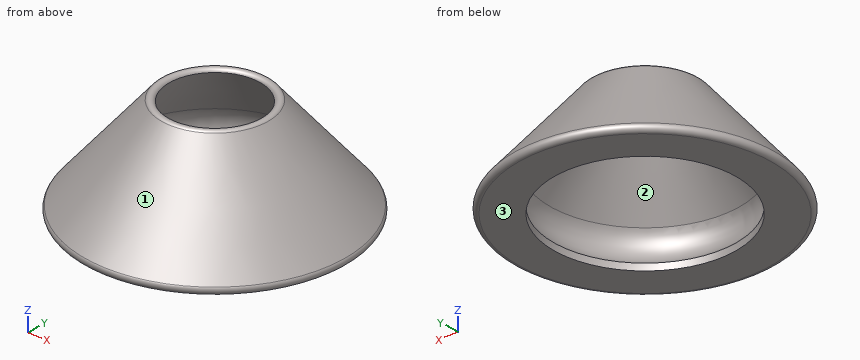
```python
from build123d import *


# Not quite as in the source:
# - a fillet or chamfer that OpenCascade refuses, or shapes differently, is made with other operations: its cross-section is extruded or revolved along the edge and cut away or added


with BuildPart() as f1:
    # F0 (on Front) → F1 (revolve)
    with BuildSketch(Plane.XZ):
        Polygon((20, 1.5), (20, 0), (30, 0), (10, 23.8350718519), (10, 21.5014861116), (26.7832396192, 1.5), align=None)
    revolve(axis=Axis((0, 0, 12.1238185093), (0, 0, 1)))

    # F2: fillet of radius 5 on 1 edges, made by hand

    # F2_s1 → F2_t2 (revolve)
    with BuildSketch(Plane.XZ):
        with BuildLine():
            ThreePointArc((20.7691072795, 8.6673638222), (21.9103444044, 4.9199541008), (20, 1.5))
            Line((20, 1.5), (20.0612222987, 1.4209314845))
            ThreePointArc((20.0612222987, 1.4209314845), (23.3916198096, 1.4), (26.7832396192, 1.4))
            Line((26.7832396192, 1.4), (26.8598440635, 1.564278761))
            Line((26.8598440635, 1.564278761), (20.8457117239, 8.7316425831))
            Line((20.8457117239, 8.7316425831), (20.7691072795, 8.6673638222))
        make_face()
    revolve(axis=Axis((0, 0, 1.5), (0, 0, 1)))

    # F3: fillet of radius 1 on 2 edges, made by hand

    # F3_s1 → F3_t2 (revolve, cut)
    with BuildSketch(Plane.XZ):
        with BuildLine():
            ThreePointArc((27.8554930795, 0), (28.7618008665, 0.5773817383), (28.6215375226, 1.6427876097))
            Line((28.6215375226, 1.6427876097), (28.6368584115, 1.6556433619))
            Line((28.6368584115, 1.6556433619), (30.0153208889, 0.0128557522))
            Line((30.0153208889, 0.0128557522), (30, -0.02))
            Line((30, -0.02), (27.8554930795, -0.02))
            Line((27.8554930795, -0.02), (27.8554930795, 0))
        make_face()
    revolve(axis=Axis((0, 0, 0), (0, 0, 1)), mode=Mode.SUBTRACT)

    # F3_s3 → F3_t4 (revolve, cut)
    with BuildSketch(Plane.XZ):
        with BuildLine():
            ThreePointArc((11.7057370639, 21.802253578), (10.7660444431, 22.1442737213), (10, 21.5014861116))
            Line((10, 21.5014861116), (9.9812061476, 21.5083265145))
            ThreePointArc((9.9812061476, 21.5083265145), (9.98, 22.6682789817), (9.98, 23.8350718519))
            Line((9.98, 23.8350718519), (10.0153208889, 23.8479276041))
            Line((10.0153208889, 23.8479276041), (11.7210579528, 21.8151093301))
            Line((11.7210579528, 21.8151093301), (11.7057370639, 21.802253578))
        make_face()
    revolve(axis=Axis((0, 0, 23.8350718519), (0, 0, 1)), mode=Mode.SUBTRACT)


solid = f1.part
```
Geometry check sheet. Reference: the model listing, model coordinates, mm. Face numbers are marked on the shaded views. Give positions to 0.01 mm unless a question says otherwise; leave off trailing zeros. Loops run counter-clockwise (first coordinate to the right, second up) from the corner with the lowest first, then second, coordinate; pieces in that order, holes last. Notation, with made-up numbers: M 56,26.5 L 85,26.5 A16 cw 85,46.5 Z; hole C -22,-2 d7. An arc over 180 degrees is marked long. Write item = value, one per line.
(1) Material ranges on line 1 (Y direction, x = -14.5, z = 1.75); line 2 (Z direction, x = 20.5, y = -6); line 3 (Y direction, x = 19.5, z = 3.25), recorded low to high. Write a range as [from, to].
Answer below:
line_1 = [-24.57, -14.2], [14.2, 24.57]
line_2 = [0, 3.12], [7.79, 10.3]
line_3 = [-19.07, -8.88], [8.88, 19.07]
(2) Sectioned sample at A-A, the plane y = 0. Record the cut outline in (x, z), plus the area to 3 significant figures.
Answer below:
outline = M -28.62,1.64 A1 ccw -27.86,0 L -20,0 L -20,1.5 A5 cw -20.77,8.67 L -10,21.5 A1 ccw -11.71,21.8 Z; M 10,21.5 L 20.77,8.67 A5 cw 20,1.5 L 20,0 L 27.86,0 A1 ccw 28.62,1.64 L 11.71,21.8 A1 ccw Z
area = 140 mm2
(3) Sectioned sample at D-D, the plane z = 10. Record the cut outline in (x, y).
Answer below:
outline = C 0,0 d43.22; hole C 0,0 d39.3
(4) Release check for a two-part mould opening along Y. For the marked faces 1, 2 and 3 record: released by +Y, released by -Y, zero draft, split by the parting line, or undercut.
Answer below:
face_1 = split by the parting line
face_2 = undercut
face_3 = zero draft
(5) Gauge pin test, flat ends, axial feed: pin 1 Ø10 at (x, z) = (1.5, 5) entering from -Y; pin 2 Ø6 at (x, z) = (-9.5, 19) entering from +Y; pin 3 Ø3 at (y, z) = (12, 10) entering from +X; pin 4 Ø10 at (x, y) = (12, 6) entering from +Z. Record the tip position at first contact, or that the pin passes through.
Answer below:
pin_1 = -28.86
pin_2 = 14.13
pin_3 = 19.72
pin_4 = 22.16
(6) Sectioned sample at C-C, the plane z = 14.5. Record the cut outline in (x, y), plus the area to 3 significant figures.
Answer below:
outline = C 0,0 d35.67; hole C 0,0 d31.75
area = 207 mm2
